Geometry: final body of the model. Coordinates: model frame, mm. A direction names the side the tool comes from. Coordinates: 2 decimals unless noted, no trailing zeros. Order: outer loops, then holes, each group sorted by start corner. A loop starts at its lowest first (then second) coordinate and runs counter-clockwise, first axis right, second up. Notation, with made-up numbers: M 28.5,55.25 L 33.5,55.25 A17 cw 33.5,70.25 Z; hole C 21,-24 d4. An arc over 180 degrees is marked long. Write item = value, one per line.
Autodesk Inventor part; units mm, degrees
ref_plane "YZ Plane" through (0, 0, 0) normal (1, 0, 0) x (0, 1, 0)
ref_plane "XZ Plane" through (0, 0, 0) normal (0, 1, 0) x (-1, 0, 0)
ref_plane "XY Plane" through (0, 0, 0) normal (0, 0, 1) x (1, 0, 0)
sketch "Эскиз4" plane through (0, 0, 0) normal (0, 0, 1) x (1, 0, 0)
  line L0 (0, 0) -> (20, 0)
  line L1 (20, 0) -> (20, 25)
  line L2 (16, 29) -> (4, 29)
  line L3 (0, 25) -> (0, 0)
  line L4 (4, 29) -> (0, 25)
  line L5 (16, 29) -> (20, 25)
  point P0 (20, 29)
  point P1 (0, 29)
  dimension "d33" = 20
  dimension "d34" = 29
  dimension "d35" = 4
  dimension "d36" = 4
  dimension "d37" = 4
  dimension "d38" = 4
revolve "Вращение3" add sketch "Эскиз4" angle 360 about axis through (0, 0, 0) along (1, 0, 0)
sketch "Эскиз5" plane through (20, 0, 0) normal (1, 0, 0) x (0, 0, -1)
  point P0 (0, 0)
  point P1 (0, 0)
hole "Отверстие2" at (20, 0, 0) direction (-1, 0, 0) diameter 12 depth 8 countersink diameter 14 countersink angle 90
sketch "Эскиз6" plane through (0, 0, 0) normal (-1, 0, 0) x (0, 0, 1)
  point P0 (0, 0)
  point P1 (0, 0)
hole "Отверстие3" at (0, 0, 0) direction (1, 0, 0) diameter 10 depth 12 countersink diameter 14 countersink angle 90
sketch "Эскиз7" plane through (0, 0, 0) normal (-1, 0, 0) x (0, 0, 1)
  line L0 (0, 0) -> (0, 23) construction
  dimension "d54" = 23
hole "Отверстие4" at (0, 23, 0) direction (1, 0, 0) diameter 4 depth 4
thread "Резьба3"
properties part number "711135"
1) Section A-A, the plane y = 0. Return loops of the section in (x, z).
Numbers:
outline = M 0,-25 L 4,-29 L 16,-29 L 20,-25 L 20,-7 L 19,-6 L 12,-6 L 12,-5 L 2,-5 L 0,-7 Z; M 0,7 L 2,5 L 12,5 L 12,6 L 19,6 L 20,7 L 20,25 L 16,29 L 4,29 L 0,25 Z
2) Pin query (flat end, axial travel): pin 1 (1.2 mm diameter, centred on y = 22.5, z = -0.5, fed in from -X); pin 2 (5 mm diameter, centred on x = 13, z = 4.5, fed in from -Y); pin 3 (6 mm diameter, centred on x = 5, y = 11.5, fed in from +Z). Return the tip coordinate at first contact, or that it passes through.
Numbers:
pin_1 = 4
pin_2 = -28.93
pin_3 = 27.73
3) Section B-B, the plane x = 8.75. Return loops of the section in (y, z), and give its area (3 significant figures).
Numbers:
outline = C 0,0 d58; hole C 0,0 d10
area = 2,560 mm²
4) Set-up query: faces 4 (the face through (2, 21, 0)), 5 (the face through (20, 5.2, -5.2)), 6 (the face through (15, 0, 6)). Return all of +Z, -Z, +X, -X, +Y, -Y with unobstructed straight access to the full face (end or side cutting, diameter ignored); none if empty.
Numbers:
face_4 = -X
face_5 = +Z, -Z, +X, +Y, -Y
face_6 = +X
5) Mould query, pull axis Y, two halves, no side actions, for faces 1 (the face through (7.07, 4.88, -1.08)), 2 (the face through (0, 5.2, -5.2)), 3 (the face through (19.75, -5.47, 24.65)). Classes: pulls with the +Y half, pulls with the -Y half, needs draft (parallel to the pull), parting line crosses it, or undercut.
Numbers:
face_1 = undercut
face_2 = needs draft
face_3 = parting line crosses it
6) Line query: L1, parallel to Z at x = 14, y = 0; L2, parallel to Y at x = 2.5, z = 0.5; L3, parallel to Z at x = 16.25, y = -4. Output: solid intervals per line, ascending.
Numbers:
L1 = -29 to -6, 6 to 29
L2 = -27.5 to -4.97, 4.97 to 21.06, 24.94 to 27.5
L3 = -28.47 to -4.47, 4.47 to 28.47
